Could you check a few things on this drawing? It's one solid part, dimensions in mm from its lowest x, y, z. A direction names the side the tool comes from. Give positions to 0.01 mm unless a question says otherwise; leave off trailing zeros. Write each loop counter-clockwise with the first axis right and the second up, starting at its lowest first coordinate (ties: lowest second). Pieces come first, ordered by that corner, then holes. Notation, with made-up numbers: (29, -18) -> (84, -18) arc R16 cw to (84, -5) -> close; hole circle Ø6 at (-29, 56). An arc over 180 degrees is marked (long way). Answer as CSV lines item,"result". Start each with the question number.
1. If we section it at B-B on z = 18: Write out the boundary of the cut face in (x, y).
2. If we section it at A-A on x = 16.5: Write out the boundary of the cut face in (y, z), plus the area to 3 significant figures.
3. If we section it at C-C on y = 7.5: Write out the boundary of the cut face in (x, z).
4. If we mould it in two halves opening along Z, with no side actions, what happens to the marked faces 1 and 2? For each: pulls with the +Z half, pulls with the -Z half, needs draft (parallel to the pull), parting line crosses it, or undercut.
5. On a 3-axis mill with a long thin cutter (end or side, diameter ignored), from which of +Z, -Z, +X, -X, +Y, -Y can I reach the whole of each face in a straight line? I mean the marked faces 3 and 4. Say none if no direction works.
6. I need wall thicknesses on line 1 (Z direction, x = 23, y = 28.5); line 2 (X direction, y = 18, z = 4) (1 decimal); line 3 (X direction, y = 22.5, z = 33.5). Which ranges of each line are inside material? Lowest first, please. Write a range as [from, to].
7. I'm going to push flat-ended pins straight in: P1, Ø5, axis at y = 7, z = 36, coming from the +X side; P2, Ø10, axis at y = 10, z = 37.5, coming from the +X side; P3, Ø2, axis at y = 21.5, z = 17.5, coming from the +X side; P4, Ø18, axis at x = 13.5, y = 24, coming from the -Z side. Where does each tip first touch, or does it pass through?
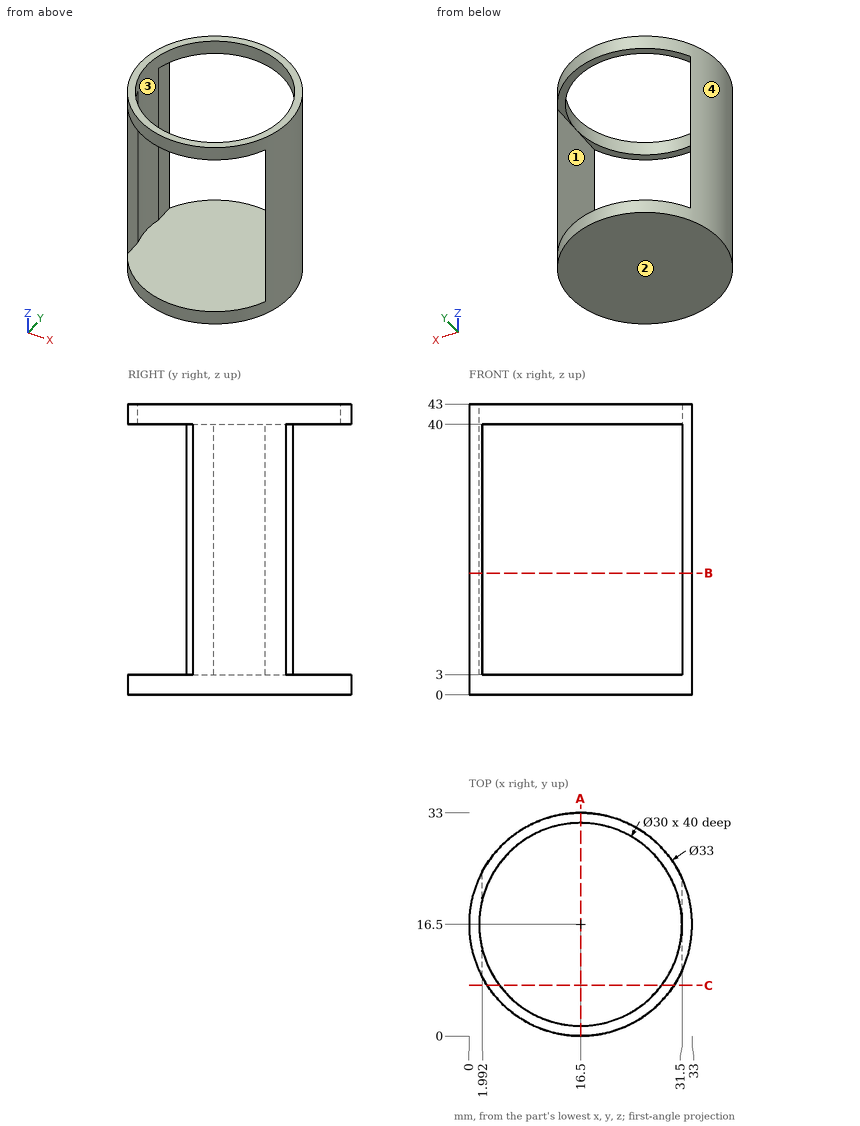
Computed values:
1,outline,"(1.99, 8.64) -> (1.99, 12.69) arc R15 cw to (1.99, 20.31) -> (1.99, 24.36) arc R16.5 ccw to start; (31.5, 9.63) arc R16.5 ccw to (31.5, 23.37) -> close"
2,outline,"(0, 0) -> (33, 0) -> (33, 3) -> (0, 3) -> close; (0, 40) -> (1.5, 40) -> (1.5, 43) -> (0, 43) -> close; (31.5, 40) -> (33, 40) -> (33, 43) -> (31.5, 43) -> close"
2,area,"108 mm2"
3,outline,"(2.67, 0) -> (30.33, 0) -> (30.33, 3) -> (2.67, 3) -> close; (2.67, 40) -> (4.5, 40) -> (4.5, 43) -> (2.67, 43) -> close; (28.5, 40) -> (30.33, 40) -> (30.33, 43) -> (28.5, 43) -> close"
4,face 1,"undercut"
4,face 2,"pulls with the -Z half"
5,face 3,"+Z"
5,face 4,"+Z, -Z"
6,line 1,"z = [0, 3]"
6,line 2,"x = [0.1, 1.6], [31.5, 32.9]"
6,line 3,"x = [1.13, 1.99], [31.5, 31.87]"
7,P1,"stops at x = 1.99"
7,P2,"stops at x = 32.93"
7,P3,"stops at x = 32.51"
7,P4,"stops at z = 0"
